Here's how the part is built. I have some questions about the finished solid (model axes, mm). A direction names the side the tool comes from. Coordinates: 2 decimals unless noted, no trailing zeros. Write each loop counter-clockwise with the first axis right and the second up, starting at its lowest first coordinate (ties: lowest second). Pieces come first, ordered by that corner, then holes.
Item 1: If we mould it in two halves opening along X, with no side actions, what happens to faces 4 (the face through (-51, 2, -20)), 5 (the face through (51, 2, -20)), 6 (the face through (47.177, 1.232, -0.256)), 7 (the face through (0.783, 1.268, -27.494))? For each: pulls with the +X half, pulls with the -X half, needs draft (parallel to the pull), parting line crosses it, or undercut.
Item 2: I'm going to push flat-ended pins straight in: P1, Ø1.5, axis at x = 28, z = -19, coming from the +Y side; P2, Ø1, axis at x = -39, y = 22, coming from the +Z side; P3, Ø6, axis at y = 4, z = -8.5, coming from the +X side; P4, Ø5, axis at x = -46, y = 15, coming from the -Z side. Where does each tip first touch, or does it pass through?
Item 3: I want a section at C-C (x = 36.5). Please give me the cut outline in (y, z), and give its area (3 significant figures).
Item 4: I want a section at A-A (y = 15). Please give me the cut outline in (x, z), and give its area (4 significant figures).
Item 5: I want a section at D-D (z = -25.25). Please give me the cut outline in (x, y).
Item 6: For faces 1 (the face through (-48.747, 15.121, -28.732)), 2 (the face through (-47.15, 1.23, -0.27)), 3 (the face through (-1, 14, -27.5)), which set-ups out of +Z, -Z, +X, -X, +Y, -Y let a thin tool reach every point of the face, with its end or its side?
Item 7: Please list where these lines run through material, in increasing order: line 1 (Y direction, x = -32, z = -25); line 2 (Z direction, x = 6, y = 5.5); line 3 (Z direction, x = 24.5, y = 2).
Item 8: I want a section at B-B (z = -17.25). Please give me the cut outline in (x, y).
Autodesk Inventor part; units mm, degrees
ref_plane "YZ Plane" through (0, 0, 0) normal (1, 0, 0) x (0, 1, 0)
ref_plane "XZ Plane" through (0, 0, 0) normal (0, 1, 0) x (-1, 0, 0)
ref_plane "XY Plane" through (0, 0, 0) normal (0, 0, 1) x (1, 0, 0)
sketch "Skizze1" plane through (0, 0, 0) normal (1, 0, 0) x (0, 1, 0)
  line L0 (0, 0) -> (0, -30)
  line L1 (0, -30) -> (25, -30)
  line L2 (25, -30) -> (25, -27.5)
  line L3 (25, -27.5) -> (2.5, -27.5)
  line L4 (2.5, -27.5) -> (2.5, 0)
  line L5 (2.5, 0) -> (0, 0)
  dimension "d0" = 30
  dimension "d1" = 25
  dimension "d2" = 2.5
  dimension "d3" = 22.5
extrude "Extrusion1" add sketch "Skizze1" along normal mid plane 102
sketch "Skizze2" plane through (-51, 2.5, 0) normal (0, 1, 0) x (1, 0, 0)
  line L0 (0, 0) -> (102, 0)
  arc A0 (98, 0) -> (4, 0) centre (51, -26.4136) ccw
  line L1 (0, 27.5) -> (102, 27.5)
  line L2 (4, 0) -> (98, 0)
  point P0 (51, 0)
  dimension "d6" = 94
extrude "Extrusion2" cut sketch "Skizze2" against normal blind 2.5
fillet "Rundung1" radius 2 4 edges at (47, 1.25, 0) (-47, 1.25, 0) (-51, 1.25, 0) (51, 1.25, 0)
sketch "Skizze3" plane through (-51, 2.5, -27.5) normal (0, 1, 0) x (1, 0, 0)
  line L0 (-0.5, 0) -> (27.5, 0) construction
  line L1 (-0.5, -28) -> (4.5665, -28)
  arc A0 (97.4335, -28) -> (4.5665, -28) centre (51, -53.8505) ccw
  line L2 (102.2546, -28) -> (97.4335, -28)
  line L3 (51, 0) -> (102, 0)
  line L4 (-0.5, -28) -> (-0.5, -23)
  arc A1 (51, 0) -> (-0.5, -23) centre (49.8083, -66.4893) ccw
  line L5 (102.2546, -28) -> (102.2546, -23)
  line L6 (102, 0) -> (102, -25.5)
  line L7 (102.2546, -28) -> (107.2546, -28) construction
  arc A2 (97.4335, -26.5163) -> (51, 0) centre (51, -53.9136) ccw
  arc A3 (102.2546, -23) -> (51, 0) centre (51.9496, -66.4932) ccw
  point P0 (51, -27.5)
  dimension "d10" = 28
  dimension "d13" = 5
  dimension "d14" = 66.5
  dimension "d20" = 5
  dimension "d21" = 90
  dimension "d22" = 66.5
extrude "Extrusion3" [suppressed]
fillet "Rundung2" [suppressed]
sketch "Skizze4" plane through (-51, 25, -27.5) normal (0, 0, 1) x (1, 0, 0)
  circle A0 centre (97, -10) radius 2.75
  circle A1 centre (5, -10) radius 2.75
  point P0 (51, -25)
  dimension "d24" = 5.5
  dimension "d25" = 5.5
extrude "Extrusion4" cut sketch "Skizze4" against normal blind 2.5
properties part number "Glashalter"
Answer:
1. face 4: pulls with the -X half
1. face 5: pulls with the +X half
1. face 6: undercut
1. face 7: undercut
2. P1: stops at y = 2.5
2. P2: stops at z = -27.5
2. P3: stops at x = 51
2. P4: passes through
3. outline: (0, -30) - (25, -30) - (25, -27.5) - (2.5, -27.5) - (2.5, -13.27) - (0, -13.27) - close
3. area: 98.1 mm2
4. outline: (-51, -30) - (-48.75, -30) - (-48.75, -27.5) - (-51, -27.5) - close; (-43.25, -30) - (43.25, -30) - (43.25, -27.5) - (-43.25, -27.5) - close; (48.75, -30) - (51, -30) - (51, -27.5) - (48.75, -27.5) - close
4. area: 227.5 mm2
5. outline: (-51, 0) - (-15.41, 0) - (-15.41, 2.5) - (-51, 2.5) - close; (15.41, 0) - (51, 0) - (51, 2.5) - (15.41, 2.5) - close
6. face 1: +Z, -Z
6. face 2: +Z, +Y, -Y
6. face 3: +Z, +X, -X, +Y
7. line 1: y = 0 to 2.5
7. line 2: z = -30 to -27.5
7. line 3: z = -30 to -21.61
8. outline: (-51, 0) - (-31.63, 0) - (-31.63, 2.5) - (-51, 2.5) - close; (31.63, 0) - (51, 0) - (51, 2.5) - (31.63, 2.5) - close
